from build123d import *

# Parameters (mm, degrees)
F0_R     = 2.75
F1_DEPTH = 3.5
F2_W     = 14.5
F2_H     = 30
F2_W_2   = 10
F2_H_2   = 3.5
F3_DEPTH = 1


with BuildPart() as f1:
    # F0 (on Front) → F1 (new body)
    with BuildSketch(Plane.XZ):
        with BuildLine():
            Line((0, 25.75), (0, 0))
            Line((0, 0), (10, 0))
            Line((10, 0), (10, 25.75))
            ThreePointArc((10, 25.75), (8.535534, 29.285534), (5, 30.75))
            ThreePointArc((5, 30.75), (1.464466, 29.285534), (0, 25.75))
        make_face()
        with Locations((5, 25.25)):
            Circle(F0_R, mode=Mode.SUBTRACT)
    extrude(amount=F1_DEPTH)

    # F2 (on face) → F3 (join)
    with BuildSketch(Plane(origin=(0, 0, 0), x_dir=(1, 0, 0), z_dir=(0, 0, -1))):
        with Locations((5, 13.5)):
            Rectangle(F2_W, F2_H)
        with Locations((5, 1.75)):
            Rectangle(F2_W_2, F2_H_2, mode=Mode.SUBTRACT)
        with Locations((5, 1.75)):
            Rectangle(F2_W_2, F2_H_2)
    extrude(amount=F3_DEPTH)

    # F4: F1 across face


with BuildPart() as f1_1:
    add(f1.part)
    add(f1.part.mirror(Plane(origin=(5, -28.5, -0.5), x_dir=(1, 0, 0), z_dir=(0, -1, 0))))


solid = f1_1.part
The listing builds one solid part. Answer for the finished solid, in the listing's coordinates (mm). A direction names the side the tool comes from. Coordinates: 2 decimals unless noted, no trailing zeros. Order: outer loops, then holes, each group sorted by start corner. A loop starts at its lowest first (then second) coordinate and runs counter-clockwise, first axis right, second up. Notation, with made-up numbers: (-15, -36.5) -> (23, -36.5) arc R37 cw to (23, 1.5) -> close; hole circle Ø10 at (-22.5, -9.5). An arc over 180 degrees is marked (long way). Answer in a Markdown table with one row per item. Add a question column.
Item 1: Find the intervals of material crossed by L1, parallel to Z at x = 5, y = -1.6; L2, parallel to Y at x = 0.75, z = 21; L3, parallel to Z at x = 7, y = -3, in increasing order. Write a range as from..to.
Item 2: Find section A-A (z = 2). Write down the section's boundary in (x, y).
Item 3: Find section B-B (x = 4.25). Write down the section's boundary in (y, z).
Item 4: Each of these flat-tipped pins is pushed along its axis until it touches: P1, Ø3, axis at x = 3, z = 19.5, coming from the -Y side; P2, Ø1.8, axis at y = -2, z = 16.5, coming from the +X side; P3, Ø3, axis at x = 5.5, z = 26, coming from the -Y side; P4, Ø4, axis at x = 10.5, y = -21.5, coming from the +Z side. Where does it stop, or does it pass through?
Item 5: Find section C-C (y = -11). Write down the section's boundary in (x, z), then the cut area to 3 significant figures.
Item 6: Determine the mould class of faces 5 (the face through (5, -28, 0)), 6 (the face through (5, -2, 28)), 7 (the face through (5, -57, 16)) for opening direction Y: +Y half, -Y half, draft (parallel to the pull), parting line (faces both ways), or undercut.
Item 7: Find section D-D (x = -0.75). Write down the section's boundary in (y, z).
Item 8: Which of the six approach directions +Z, -Z, +X, -X, +Y, -Y give full straight-line access (tool end or side, diameter ignored) to faces 1 (the face through (5, 0, 16)), 2 (the face through (0, -55, 13)), 3 (the face through (5, -53.5, 16)), 4 (the face through (10, -55, 13))?
Result set:
| question | item | result |
|---|---|---|
| 1 | L1 | z = -1..22.5, 28..30.75 |
| 1 | L2 | y = -57..-53.5, -3.5..0 |
| 1 | L3 | z = -1..23.36, 27.14..30.33 |
| 2 | outline | (0, -57) -> (10, -57) -> (10, -53.5) -> (0, -53.5) -> close; (0, -3.5) -> (10, -3.5) -> (10, 0) -> (0, 0) -> close |
| 3 | outline | (-58.5, -1) -> (1.5, -1) -> (1.5, 0) -> (0, 0) -> (0, 22.6) -> (-3.5, 22.6) -> (-3.5, 0) -> (-53.5, 0) -> (-53.5, 22.6) -> (-57, 22.6) -> (-57, 0) -> (-58.5, 0) -> close; (-57, 27.9) -> (-53.5, 27.9) -> (-53.5, 30.69) -> (-57, 30.69) -> close; (-3.5, 27.9) -> (0, 27.9) -> (0, 30.69) -> (-3.5, 30.69) -> close |
| 4 | P1 | stops at y = -57 |
| 4 | P2 | stops at x = 10 |
| 4 | P3 | passes through |
| 4 | P4 | stops at z = 0 |
| 5 | outline | (-2.25, -1) -> (12.25, -1) -> (12.25, 0) -> (-2.25, 0) -> close |
| 5 | area | 14.5 mm² |
| 6 | face 5 | undercut |
| 6 | face 6 | draft |
| 6 | face 7 | -Y half |
| 7 | outline | (-58.5, -1) -> (1.5, -1) -> (1.5, 0) -> (-58.5, 0) -> close |
| 8 | face 1 | +Z, +X, -X, +Y |
| 8 | face 2 | +Z, -X, +Y, -Y |
| 8 | face 3 | +Z, +X, -X |
| 8 | face 4 | +Z, +X, +Y, -Y |
